from build123d import *

# Parameters (mm, degrees)
F3_R     = 7.2
F4_DEPTH = 3
F5_SIZE2 = 0.75
F5_SIZE  = 1.2990381057


with BuildPart() as f2:
    # F0 (on Right) → F2 (revolve)
    with BuildSketch(Plane.YZ):
        Polygon((0, 6), (0, 0), (60, 0), (60, 4.4), (57.5712198913, 5.25), (50.5712198913, 5.25), (50.5712198913, 4.4), (43.6577536166, 4.4), (38.5712198913, 5.25), (36.8757098913, 5.25), (27.7, 7), (25.5, 7), (25.5, 7.2), (15, 7.2), (15, 6), align=None)
    revolve(axis=Axis((0, -0.2503991127, 0), (0, 1, 0)))

    # F3 (on face) → F4 (join)
    with BuildSketch(Plane.XZ.offset(-15)):
        Polygon((5.1961524227, 9), (-5.1961524227, 9), (-10.3923048454, 0), (-5.1961524227, -9), (5.1961524227, -9), (10.3923048454, 0), align=None)
        Circle(F3_R, mode=Mode.SUBTRACT)
    extrude(amount=-F4_DEPTH)

    # F5
    f5_edges = [f2.edges().sort_by_distance(p)[0] for p in [
        (0, 0, -6),
    ]]
    f5_side = f2.faces().sort_by_distance((0, 7.5, -6))[0]
    chamfer(f5_edges, length=F5_SIZE, length2=F5_SIZE2, reference=f5_side)


solid = f2.part
Geometry: final body of the model. Coordinates: model frame, mm. A direction names the side the tool comes from. Coordinates: 2 decimals unless noted, no trailing zeros. Order: outer loops, then holes, each group sorted by start corner. A loop starts at its lowest first (then second) coordinate and runs counter-clockwise, first axis right, second up.
(1) Access query for faces 4 (the face through (7.76, 16.48, -4.56)), 5 (the face through (0, 8, -6)), 6 (the face through (1.6, 37.7, 5)), 7 (the face through (-4.624, 41.644, -1.027)). Directions: +Z, -Z, +X, -X, +Y, -Y. A direction counts if a zero-diameter tool reaches every point of the face in a straight line with its end or side. Return the directions, or none.
(2) Draft query along Y for faces 1 (the face through (7.83, 16.48, 4.44)), 2 (the face through (-3, 50.571, -4)), 3 (the face through (2, 15, 6)). Return one class per face: pulls with the +Y half, pulls with the -Y half, needs draft (parallel to the pull), parting line crosses it, or undercut.
(3) First-contact query: pin 1 (3 mm diameter, centred on y = 42.5, z = 2.5, fed in from -X); pin 2 (4 mm diameter, centred on y = 44, z = -6, fed in from +X); pin 3 (2 mm diameter, centred on y = 19.5, z = -3.5, fed in from -X). Flat tips, straight axial feed; report the tip coordinate or a pass-through.
(4) Material intervals for probe 1 along Y at (x, z) = (1.75, -7.5); probe 2 along Y at (x, z) = (5.75, -4.25); probe 3 along X at (y, z) = (20, 4), sorted ascending.
(5) Section query C-C (y = 40). Return the cut outline in (x, z), plus the area to 3 significant figures.
(6) Section query B-B (y = 4). Return the cut outline in (x, z), plus the area to 3 significant figures.
(7) Section query D-D (x = 9.25). Return the cut outline in (y, z), plus the area to 3 significant figures.
Solution:
1. face 4: -Z, +X, +Y, -Y
1. face 5: -Y
1. face 6: +Y
1. face 7: none
2. face 1: needs draft
2. face 2: undercut
2. face 3: pulls with the -Y half
3. pin 1: stops at x = -4.56
3. pin 2: stops at x = 1.83
3. pin 3: stops at x = -6.75
4. probe 1: y = 15 to 18
4. probe 2: y = 15 to 25.5
4. probe 3: x = -5.99 to 5.99
5. outline: circle Ø10.02 at (0, 0)
5. area: 78.9 mm2
6. outline: circle Ø12 at (0, 0)
6. area: 113 mm2
7. outline: (15, -1.98) - (18, -1.98) - (18, 1.98) - (15, 1.98) - close
7. area: 11.9 mm2
